```python
from build123d import *

# Parameters (mm, degrees)
ESBO_O4_W                        = 2.25
ESBO_O4_H                        = 16
F_4_5_4_5_DIAMETER_HOLE2_D       = 4.5
F_4_5_4_5_DIAMETER_HOLE2_DEPTH   = 18
F_4_5_4_5_DIAMETER_HOLE2_TIP     = 1.351936393
ESBO_O12_R                       = 16
ESBO_O12_R_2                     = 9
RESSALTO_EXTRUS_O1_DEPTH         = 1
CHANFRO1_SIZE                    = 0.5
CHANFRO2_SIZE                    = 0.25
FURO_DE_DI_METRO_4_5_4_5_2_D     = 4.5
FURO_DE_DI_METRO_4_5_4_5_2_DEPTH = 8
FURO_DE_DI_METRO_4_5_4_5_2_TIP   = 1.351936393
CORTE_EXTRUS_O4_START            = -0.5
ESBO_O18_R                       = 4
ESBO_O18_R_2                     = 2.25
CORTE_EXTRUS_O4_DEPTH            = 0.5
PADR_OCIRCULAR6_COUNT            = 2
PADR_OCIRCULAR6_ANGLE            = 30
PADR_OCIRCULAR7_COUNT            = 2
PADR_OCIRCULAR7_ANGLE            = 210
REBAIXO_INSERTO_REACH            = 29.148
ESBO_O20_R                       = 10


# Read off the part's stored shape, not the designer's step: PadrãoCircular5
with BuildPart() as part:
    # Esboço1 → Revolução1 (revolve)
    with BuildSketch(Plane.XY, mode=Mode.PRIVATE) as revolu_o1_sk:
        Polygon((3, -9), (16, -9), (16, 5), (9, 5), (9, -5), (3, -5), align=None)
    revolve(revolu_o1_sk.sketch.rotate(Axis((0, -9, 0), (0, 1, 0)), 90), axis=Axis((0, -9, 0), (0, 1, 0)))

    # Esboço4 → Furo de diâmetro Ø4.5 (4.5)1 (revolve, cut)
    with BuildSketch(Plane(origin=(16, 0, 0), x_dir=(0, 0, -1), z_dir=(0, 1, 0))):
        with Locations((1.125, 8)):
            Rectangle(ESBO_O4_W, ESBO_O4_H)
    revolve(axis=Axis((22.35, 0, 0), (-1, 0, 0)), mode=Mode.SUBTRACT)

    # Ø4.5 (4.5) Diameter Hole2
    with Locations(Plane(origin=(-13.856406461, 0, -8), x_dir=(0, -1, 0), z_dir=(-0.8660254037844364, 0, -0.5000000000000041))):
        with Locations((0, 0)):
            Hole(F_4_5_4_5_DIAMETER_HOLE2_D / 2, depth=F_4_5_4_5_DIAMETER_HOLE2_DEPTH)
            with Locations((0, 0, -(F_4_5_4_5_DIAMETER_HOLE2_DEPTH + F_4_5_4_5_DIAMETER_HOLE2_TIP / 2))):  # 118° drill point
                Cone(0, F_4_5_4_5_DIAMETER_HOLE2_D / 2, F_4_5_4_5_DIAMETER_HOLE2_TIP, mode=Mode.SUBTRACT)

    # Esboço12 → Ressalto-extrusão1 (add)
    with BuildSketch(Plane(origin=(0, 5, 0), x_dir=(1, 0, 0), z_dir=(0, 1, 0))):
        with Locations(Location((0, 0, 0), (0, 0, 90))):
            Circle(ESBO_O12_R)
        with Locations(Location((0, 0, 0), (0, 0, 90))):
            Circle(ESBO_O12_R_2, mode=Mode.SUBTRACT)
    extrude(amount=RESSALTO_EXTRUS_O1_DEPTH)

    # Esboço13 → Furo roscado de M3x0.51 (revolve, cut)
    with BuildSketch(Plane(origin=(11.328847338, 6, -5.282728272), x_dir=(0, 0, 1), z_dir=(1, 0, 0))):
        Polygon((0, 0), (0, 10.751075774), (1.25, 10), (1.25, 0), align=None)
    revolve(axis=Axis((11.328847338, 12.35, -5.282728272), (0, -1, 0)), mode=Mode.SUBTRACT)

    # PadrãoCircular5 outline → PadrãoCircular5 (revolve, cut)
    with BuildSketch(Plane(origin=(5.282728272, 0, 11.328847338), x_dir=(1, 0, 0), z_dir=(0, 0, 1))):
        Polygon((0, 6), (0, -4.751075774), (1.25, -4), (1.25, 6), align=None)
    revolve(axis=Axis((5.282728272, 0, 11.328847338), (0, 1, 0)), mode=Mode.SUBTRACT)

    # Padr_oCircular5 2 outline → Padr_oCircular5 2 (revolve, cut)
    with BuildSketch(Plane(origin=(-11.328847338, 0, 5.282728272), x_dir=(1, 0, 0), z_dir=(0, 0, 1))):
        Polygon((0, 6), (0, -4.751075774), (1.25, -4), (1.25, 6), align=None)
    revolve(axis=Axis((-11.328847338, 0, 5.282728272), (0, 1, 0)), mode=Mode.SUBTRACT)

    # Padr_oCircular5 3 outline → Padr_oCircular5 3 (revolve, cut)
    with BuildSketch(Plane(origin=(-5.282728272, 0, -11.328847338), x_dir=(1, 0, 0), z_dir=(0, 0, 1))):
        Polygon((0, 6), (0, -4.751075774), (1.25, -4), (1.25, 6), align=None)
    revolve(axis=Axis((-5.282728272, 0, -11.328847338), (0, 1, 0)), mode=Mode.SUBTRACT)

    # Chanfro1
    chanfro1_edges = [part.edges().sort_by_distance(p)[0] for p in [
        (0, -5, 3),
    ]]
    chamfer(chanfro1_edges, length=CHANFRO1_SIZE)

    # Chanfro2
    chanfro2_edges = [part.edges().sort_by_distance(p)[0] for p in [
        (0, 6, 9),
    ]]
    chamfer(chanfro2_edges, length=CHANFRO2_SIZE)

    # Furo de diâmetro Ø4.5 (4.5)2
    with Locations(Plane(origin=(-16, 0, 0), x_dir=(0, 0, -1), z_dir=(-1, 0, 0))):
        with Locations((0, 0)):
            Hole(FURO_DE_DI_METRO_4_5_4_5_2_D / 2, depth=FURO_DE_DI_METRO_4_5_4_5_2_DEPTH)
            with Locations((0, 0, -(FURO_DE_DI_METRO_4_5_4_5_2_DEPTH + FURO_DE_DI_METRO_4_5_4_5_2_TIP / 2))):  # 118° drill point
                Cone(0, FURO_DE_DI_METRO_4_5_4_5_2_D / 2, FURO_DE_DI_METRO_4_5_4_5_2_TIP, mode=Mode.SUBTRACT)

    # Esboço18 → Corte-extrusão4 (cut)
    with BuildSketch(Plane(origin=(-13.856406461, 0, -8), x_dir=(0, -1, 0), z_dir=(-0.8660254037844364, 0, -0.5000000000000041)).offset(CORTE_EXTRUS_O4_START)):
        Circle(ESBO_O18_R)
        with Locations(Location((0, 0, 0), (0, 0, 90))):
            Circle(ESBO_O18_R_2, mode=Mode.SUBTRACT)
    corte_extrus_o4 = extrude(amount=CORTE_EXTRUS_O4_DEPTH, mode=Mode.SUBTRACT)

    # PadrãoCircular6: Corte-extrusão4 ×2 about axis
    padr_ocircular6_axis = Axis((0, -9.75, 0), (0, 1, 0))
    for i in range(1, PADR_OCIRCULAR6_COUNT):
        add(corte_extrus_o4.rotate(padr_ocircular6_axis, i * PADR_OCIRCULAR6_ANGLE / (PADR_OCIRCULAR6_COUNT - 1)), mode=Mode.SUBTRACT)

    # PadrãoCircular7: Corte-extrusão4 ×2 about axis
    padr_ocircular7_axis = Axis((0, -9.75, 0), (0, 1, 0))
    for i in range(1, PADR_OCIRCULAR7_COUNT):
        add(corte_extrus_o4.rotate(padr_ocircular7_axis, i * PADR_OCIRCULAR7_ANGLE / (PADR_OCIRCULAR7_COUNT - 1)), mode=Mode.SUBTRACT)

    # Rebaixo_Inserto: up to this face of the body (flat: up to its plane)
    rebaixo_inserto_end = Plane(part.part.faces().sort_by_distance((0, -5, 3.754558441))[0])
    # Esboço20 → Rebaixo_Inserto (cut, up to the picked face)
    with BuildSketch(Plane(origin=(0, 6, 0), x_dir=(1, 0, 0), z_dir=(0, 1, 0)), mode=Mode.PRIVATE) as rebaixo_inserto_sk1:
        with Locations(Location((0, 0, 0), (0, 0, 270))):
            Circle(ESBO_O20_R)
    rebaixo_inserto_tool1 = split(extrude(rebaixo_inserto_sk1.sketch, amount=-REBAIXO_INSERTO_REACH, mode=Mode.PRIVATE), bisect_by=rebaixo_inserto_end, keep=Keep.BOTH, mode=Mode.PRIVATE)
    add(rebaixo_inserto_tool1.solids().sort_by(Axis((0, 6, 0), (0, -1, 0)))[0], mode=Mode.SUBTRACT)


solid = part.part
```
Input: part model. Units: mm. Frame: model coordinates. A direction names the side the tool comes from. Round coordinates to 2 decimals unless told otherwise and drop trailing zeros. Loops run counter-clockwise (first coordinate to the right, second up) from the corner with the lowest first, then second, coordinate; pieces in that order, holes last. Notation, with made-up numbers: M -22,5.5 L 14,5.5 A21 ccw 14,20.5 Z; hole C 31.5,-39 d7. An arc over 180 degrees is marked long. Answer in a Markdown table with one row per item. Add a question column.
1. Section A-A (x = 0). Output: boundary loops of the cut face in (y, z), and give its area (3 significant figures).
2. Ray query, probe 1 along X at (y, z) = (-2.5, 0); probe 2 along X at (y, z) = (-8.2, 0); probe 3 along Z at (x, y) = (8.5, 5). Return the intervals inside material, ascending.
3. Mould query, pull axis Z, two halves, no side actions, for faces 1 (the face through (-11.23, 2.15, -5.71)), 2 (the face through (-0.2, -9, 3.3)), 3 (the face through (15.62, -3.06, 3.47)). Classes: released by +Z, released by -Z, zero draft, split by the parting line, or undercut.
4. Section D-D (y = -3.5). Output: boundary loops of the cut face in (x, z).
5. Section B-B (z = 0). Give the number of separate pieces and of enclosed holes in the cut face, and give its area (3 significant figures).
6. Contact query for flat-ended pins moving along their axis: pin 1 (6 mm diameter, centred on x = -4, z = -3.5, fed in from +Y); pin 2 (1.5 mm diameter, centred on x = 5.28, z = 11.33, fed in from +Y); pin 3 (5 mm diameter, centred on x = 12, y = 2, fed in from -Z). Output: stop coordinate, or through.
7. Set-up query: faces 4 (the face through (15.5, -2, 2)), 5 (the face through (10.4, 6, 0.2)), 6 (the face through (-15.5, -2, -2)), 7 (the face through (-5.554, 1.07, -10.109)), 8 (the face through (-13.55, -4, -7.92)). Return all of +Z, -Z, +X, -X, +Y, -Y with unobstructed straight access to the full face (end or side cutting, diameter ignored); none if empty.
8. Section C-C (y = 0). Output: boundary loops of the cut face in (x, z), and give its area (3 significant figures).
Values follow:
| question | item | result |
|---|---|---|
| 1 | outline | M -9,-16 L 6,-16 L 6,-10 L -5,-10 L -5,-3.5 L -5.5,-3 L -9,-3 Z; M -9,3 L -5.5,3 L -5,3.5 L -5,10 L 6,10 L 6,16 L -9,16 Z |
| 1 | area | 236 mm^2 |
| 2 | probe 1 | -15.5 to -10, 10 to 15.5 |
| 2 | probe 2 | -16 to -3, 3 to 16 |
| 2 | probe 3 | -13.56 to -5.27, 5.27 to 13.56 |
| 3 | face 1 | undercut |
| 3 | face 2 | zero draft |
| 3 | face 3 | split by the parting line |
| 4 | outline | M -15.88,-1.94 A16 ccw -14.72,-6.26 L -14.39,-6.07 L -12.46,-9.43 L -12.79,-9.62 A16 ccw 15.88,-1.94 L 15.5,-1.94 L 15.5,1.94 L 15.88,1.94 A16 ccw -15.88,1.94 L -15.5,1.94 L -15.5,-1.94 Z; hole C -11.33,5.28 d2.5; hole C 0,0 d20; hole C -5.28,-11.33 d2.5; hole C 5.28,11.33 d2.5; hole C 11.33,-5.28 d2.5 |
| 5 | separate pieces | 4 |
| 5 | enclosed holes | 0 |
| 5 | area | 178 mm^2 |
| 6 | pin 1 | y = -5 |
| 6 | pin 2 | y = -4.3 |
| 6 | pin 3 | z = -12.87 |
| 7 | face 4 | +X |
| 7 | face 5 | +Z, -Z, +X, -X, +Y |
| 7 | face 6 | -X |
| 7 | face 7 | +Y |
| 7 | face 8 | none |
| 8 | outline | M -15.5,-3.97 A16 ccw -15.41,-4.31 L -14.55,-5.8 L -9.56,-2.92 A10 cw -9.74,-2.25 L -15.5,-2.25 Z; M -15.5,2.25 L -9.74,2.25 A10 cw 9.74,2.25 L 15.5,2.25 L 15.5,3.97 A16 ccw -15.5,3.97 Z; M -12.3,-9.7 L -11.44,-11.19 A16 ccw 15.5,-3.97 L 15.5,-2.25 L 9.74,-2.25 A10 cw -7.31,-6.82 Z; hole C -11.33,5.28 d2.5; hole C -5.28,-11.33 d2.5; hole C 5.28,11.33 d2.5; hole C 11.33,-5.28 d2.5 |
| 8 | area | 387 mm^2 |
